Here's how the part is built. I have some questions about the finished solid (model axes, mm). Give positions to 0.01 mm unless a question says otherwise; leave off trailing zeros. Write each loop counter-clockwise with the first axis right and the second up, starting at its lowest first coordinate (ties: lowest second). Pieces come first, ordered by that corner, then holes. Notation, with made-up numbers: (25, -31) - (84, -31) arc R13 ccw to (84, -6) - close; hole circle Ø2 at (13.25, 79). An arc over 180 degrees is marked (long way). Write each question's results on one line, items separated by ' | '. Start each with the question number.
Item 1: Suppose I cut it at A-A on x = 0. List the corners of the cut face in (y, z) for me (3 decimals).
Item 2: Suppose I cut it at B-B on y = -0.4. List the corners of the cut face in (x, z) for me (1 decimal), then the cut area to 3 significant figures.
Item 3: Please list where these lines run through material, in increasing order: line 1 along Z through (x, y) = (0, -0.2); line 2 along Z through (x, y) = (-0.65, 0.3).
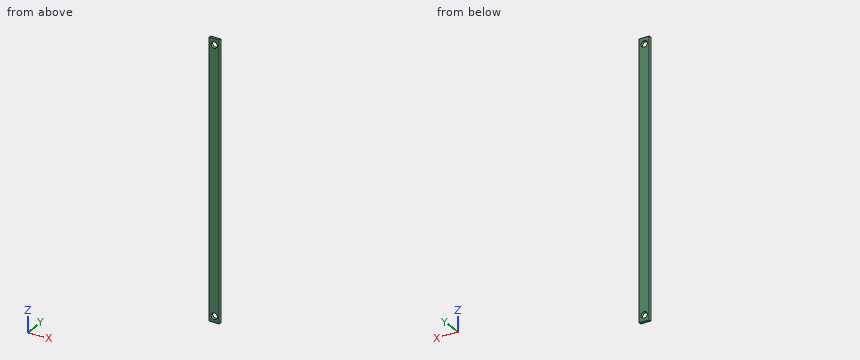
Autodesk Inventor part; units mm, degrees
ref_plane "Work Plane1" through (0, 0, 59.69) normal (0, 0, 1) x (1, 0, 0)
ref_plane "YZ Plane" through (0, 0, 0) normal (1, 0, 0) x (0, 1, 0)
ref_plane "XZ Plane" through (0, 0, 0) normal (0, 1, 0) x (-1, 0, 0)
sketch "Sketch1" plane through (0, 0, 0) normal (0, 0, 1) x (1, 0, 0)
  line L0 (2.54, -0.635) -> (-2.54, -0.635)
  line L1 (-2.54, -0.635) -> (-2.54, 0.635)
  line L2 (-2.54, 0.635) -> (2.54, 0.635)
  line L3 (2.54, 0.635) -> (2.54, -0.635)
  line L4 (2.54, -0.635) -> (-2.54, 0.635) construction
  line L5 (-2.54, -0.635) -> (2.54, 0.635) construction
  point P0 (0, 0)
  dimension "d0" = 5.08
  dimension "d1" = 1.27
extrude "Extrusion1" add sketch "Sketch1" along normal blind 119.38
ref_plane "Work Plane1" through (0, 0, 59.69) normal (0, 0, 1) x (1, 0, 0)
sketch "Sketch2" plane through (0, 0, 119.38) normal (0, 0, 1) x (1, 0, 0)
  line L0 (2.54, 0.635) -> (-2.54, 0.635)
  line L1 (-2.54, 0.635) -> (-2.54, -0.635)
  line L2 (-2.54, -0.635) -> (2.54, -0.635)
  line L3 (2.54, -0.635) -> (2.54, 0.635)
  point P0 (0, 0)
extrude "Extrusion2" add sketch "Sketch2" along normal blind 10.16
sketch "Sketch3" plane through (-2.54, 0.635, 0) normal (0, 1, 0) x (1, 0, 0)
  line L0 (5.08, -119.38) -> (0, -119.38) construction
  line L1 (2.54, -119.38) -> (2.54, -129.54) construction
  line L2 (0, -129.54) -> (5.08, -129.54) construction
  circle A0 centre (2.54, -126.3807) radius 1.5875
  point P0 (2.54, 0)
extrude "Extrusion3" cut sketch "Sketch3" against normal blind 6.35
mirror "Mirror1" about plane through (0, 0, 59.69) normal (0, 0, 1) of "Extrusion2"
mirror "Mirror2" about plane through (0, 0, 59.69) normal (0, 0, 1) of "Extrusion3"
thread "Thread1"
thread "Thread2"
properties part number "Pedal Bar"
Checked values:
1) outline: (-0.635, -10.16) - (0.635, -10.16) - (0.635, -8.588) - (-0.635, -8.588) - close; (-0.635, -5.413) - (0.635, -5.413) - (0.635, 124.793) - (-0.635, 124.793) - close; (-0.635, 127.968) - (0.635, 127.968) - (0.635, 129.54) - (-0.635, 129.54) - close
2) outline: (-2.5, -10.2) - (2.5, -10.2) - (2.5, 129.5) - (-2.5, 129.5) - close; hole circle Ø3.2 at (0, -7); hole circle Ø3.2 at (0, 126.4) | area: 694 mm^2
3) line 1: z = -10.16 to -8.59, -5.41 to 124.79, 127.97 to 129.54 | line 2: z = -10.16 to -8.45, -5.55 to 124.93, 127.83 to 129.54
